Autodesk Inventor part; units mm, degrees
ref_plane "YZ Plane" through (0, 0, 0) normal (1, 0, 0) x (0, 1, 0)
ref_plane "XZ Plane" through (0, 0, 0) normal (0, 1, 0) x (-1, 0, 0)
ref_plane "XY Plane" through (0, 0, 0) normal (0, 0, 1) x (1, 0, 0)
sketch "Szkic1" plane through (0, 0, 0) normal (0, 1, 0) x (-1, 0, 0)
  line L0 (9.5668, 14.1781) -> (9.5668, 20.6781)
  line L1 (15.0668, 14.1781) -> (9.5668, 14.1781)
  arc A0 (15.0668, 14.1781) -> (15.0668, 20.6781) centre (15.0668, 17.4281) ccw
  line L2 (9.5668, 20.6781) -> (15.0668, 20.6781)
  circle A1 centre (15.0668, 17.4281) radius 1.6
  line L3 (-14.9332, 20.6781) -> (-9.4332, 20.6781)
  arc A2 (-14.9332, 20.6781) -> (-14.9332, 14.1781) centre (-14.9332, 17.4281) ccw
  line L4 (-9.4332, 14.1781) -> (-14.9332, 14.1781)
  line L5 (-9.4332, 20.6781) -> (-9.4332, 14.1781)
  circle A3 centre (-14.9332, 17.4281) radius 1.6
  point P0 (0, 0)
extrude "Wyciągnięcie proste1" add sketch "Szkic1" along normal blind 3.15
sketch "Szkic2" plane through (0, 3.15, 0) normal (0, 1, 0) x (1, 0, 0)
  line L0 (-9.5668, -20.6781) -> (-9.5668, -14.1781)
  line L1 (9.4332, -14.1781) -> (9.4332, -20.6781)
  line L2 (-15.0668, -20.6781) -> (-9.5668, -20.6781)
  line L3 (9.4332, -14.1781) -> (9.4332, -20.6781)
  line L4 (-9.5668, -20.6781) -> (9.4332, -20.6781)
  line L5 (-9.5668, -14.1781) -> (-15.0668, -14.1781)
  line L6 (9.4332, -14.1781) -> (-9.5668, -14.1781)
  point P0 (0, 0)
extrude "Wyciągnięcie proste2" add sketch "Szkic2" against normal blind 1
fillet "Zaokrąglenie1" radius 0.8 2 edges at (9.4332, 2.15, 17.4281) (-9.5668, 2.15, 17.4281)
fillet "Zaokrąglenie2" radius 0.5 6 edges at (9.4332, 0.675, 14.1781) (-9.5668, 0.675, 14.1781) (-0.0668, 2.15, 14.1781) (-9.5668, 0.675, 20.6781) (9.4332, 0.675, 20.6781) (-0.0668, 2.15, 20.6781)
properties part number "dol_trzymacz"
Work out the finished part from the listing and answer in its coordinate system (mm). A direction names the side the tool comes from. Give positions to 0.01 mm unless a question says otherwise; leave off trailing zeros. Order: outer loops, then holes, each group sorted by start corner. A loop starts at its lowest first (then second) coordinate and runs counter-clockwise, first axis right, second up. Notation, with made-up numbers: (-30.5, 7.25) -> (-0.5, 7.25) arc R28 ccw to (-0.5, 40.25) -> close; hole circle Ø1 at (-25, 67). An arc over 180 degrees is marked (long way). Answer as CSV lines item,"result". Start each with the question number.
(1) Each of these flat-tipped pins is pushed along its axis until it touches: pin 1 Ø1.5 at (y, z) = (0.5, 16) entering from +X; pin 2 Ø3 at (x, z) = (-3.5, 17) entering from -Y; pin 3 Ø1 at (y, z) = (0.5, 18.5) entering from -X. Where does it stop, or does it pass through?
(2) Section B-B, the plane z = 16.25 is taken. Write down the section's boundary in (x, y).
(3) Section D-D, the plane y = 1.85 is taken. Give the number of separate pieces and of enclosed holes in the cut face, plus the area to 3 significant figures.
(4) Section A-A, the plane y = 0.3 is taken. Write down the section's boundary in (x, z), plus the area to 3 significant figures.
(5) Consider line 1 along X through (y, z) = (0.8, 16.25); line 2 along Y through (x, z) = (-5, 15.25); line 3 along X through (y, z) = (0.4, 15.75). Determine where each line is inside the solid, lowest interval first.
(6) Section C-C, the plane x = -2.5 is taken. Write down the section's boundary in (y, z).
(7) For a pull along X with two mould halves and no side action, classify faces 3 (the flat face through (13, 0, 17)), 4 (the cylindrical face through (18.182, 1.553, 17.357)), 5 (the flat face through (9.433, 1, 17)) as released by +X, released by -X, zero draft, split by the parting line, or undercut.
(8) Which of the six approach directions +Z, -Z, +X, -X, +Y, -Y give full straight-line access (tool end or side, diameter ignored) to faces 1 (the flat face through (0, 3.15, 17)), 2 (the flat face through (0, 2.15, 17))?
Entries:
1,pin 1,"x = 18.11"
1,pin 2,"y = 2.15"
1,pin 3,"x = -18.27"
2,outline,"(-18.1, 0) -> (-16.15, 0) -> (-16.15, 3.15) -> (-18.1, 3.15) -> close; (-13.98, 0) -> (-9.57, 0) -> (-9.57, 1.35) arc R0.8 cw to (-8.77, 2.15) -> (8.63, 2.15) arc R0.8 cw to (9.43, 1.35) -> (9.43, 0) -> (13.85, 0) -> (13.85, 3.15) -> (-13.98, 3.15) -> close; (16.02, 0) -> (17.96, 0) -> (17.96, 3.15) -> (16.02, 3.15) -> close"
3,separate pieces,"2"
3,enclosed holes,"2"
3,area,"90.6 mm²"
4,outline,"(-15.07, 14.18) -> (-10.07, 14.18) arc R0.5 ccw to (-9.57, 14.68) -> (-9.57, 20.18) arc R0.5 ccw to (-10.07, 20.68) -> (-15.07, 20.68) arc R3.25 ccw to start; (9.43, 14.68) arc R0.5 ccw to (9.93, 14.18) -> (14.93, 14.18) arc R3.25 ccw to (14.93, 20.68) -> (9.93, 20.68) arc R0.5 ccw to (9.43, 20.18) -> close; hole circle Ø3.2 at (-15.07, 17.43); hole circle Ø3.2 at (14.93, 17.43)"
4,area,"88.4 mm²"
5,line 1,"-18.1 to -16.15, -13.98 to -9.57, 9.43 to 13.85, 16.02 to 17.96"
5,line 2,"2.15 to 3.15"
5,line 3,"-17.85 to -9.57, 9.43 to 17.72"
6,outline,"(2.15, 14.68) arc R0.5 ccw to (2.65, 14.18) -> (3.15, 14.18) -> (3.15, 20.68) -> (2.65, 20.68) arc R0.5 ccw to (2.15, 20.18) -> close"
7,face 3,"zero draft"
7,face 4,"released by +X"
7,face 5,"undercut"
8,face 1,"+Z, -Z, +X, -X, +Y"
8,face 2,"+Z, -Z, -Y"
